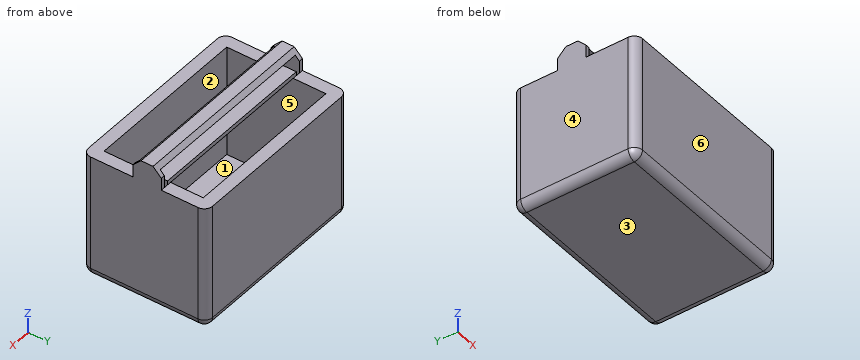
```python
from build123d import *

# Parameters (mm, degrees)
F0_W         = 116.5109202266
F0_H         = 75.9218987077
F1_DEPTH     = 76.2
F2_T         = -7.62
F3_W         = 116.5109202266
F3_H         = 17.5204388797
F4_DEPTH     = 12.7
F5_T         = -2.54
F6_R         = 5.08
F7_R         = 5.08
F8_R         = 5.08
F9_T1_DEPTH  = 66.04
F9_T3_DEPTH  = 106.3509202266
F9_T5_DEPTH  = 83.5418987077
F9_S9_W      = 5.08
F9_S9_H      = 5.08
F9_T10_DEPTH = 5.08
F9_T14_ANGLE = 90
F9_T16_ANGLE = 90
F10_T1_DEPTH = 142.6392193843
F11_T1_DEPTH = 142.6392193843


# Not quite as in the source:
# - a fillet or chamfer that OpenCascade refuses, or shapes differently, is made with other operations: its cross-section is extruded or revolved along the edge and cut away or added
# - a shell that OpenCascade refuses in one call is made with other operations: the cavity is built on its own and cut out


with BuildPart() as f1:
    # F0 (on Front) → F1 (new body)
    with BuildSketch(Plane.XZ):
        with Locations((6.8621747196, 17.2284292057)):
            Rectangle(F0_W, F0_H)
    extrude(amount=F1_DEPTH)

    # F2
    f2_openings = [f1.faces().sort_by_distance(p)[0] for p in [
        (6.862175, -38.1, 55.189379),
    ]]
    offset(amount=F2_T, openings=f2_openings)

    # F3 (on face) → F4 (join)
    with BuildSketch(Plane.XY.offset(55.1893785596)):
        with Locations((6.8621747196, -36.5009140223)):
            Rectangle(F3_W, F3_H)
    extrude(amount=F4_DEPTH)

    # F5: a shell. OpenCascade refuses it in one call, so the cavity is built on its own and cut out:
    # the body offset inwards by the wall thickness, plus a prism from it out through each open face.
    f5_core = offset(f1.part, amount=F5_T, kind=Kind.INTERSECTION, mode=Mode.PRIVATE)
    f5_exits = [f5_core.faces().sort_by_distance(p)[0] for p in [
        (6.862175, -42.721133, 61.352079),
        (6.862175, -30.280695, 61.352079),
    ]]
    add(f5_core, mode=Mode.SUBTRACT)
    extrude(f5_exits, amount=-F5_T, mode=Mode.SUBTRACT)

    # F6
    f6_edges = [f1.edges().sort_by_distance(p)[0] for p in [
        (65.117635, 0, 17.228429),
    ]]
    fillet(f6_edges, radius=F6_R)

    # F7
    f7_edges = [f1.edges().sort_by_distance(p)[0] for p in [
        (4.322175, 0, -20.73252),
        (-51.393285, 0, 17.228429),
    ]]
    fillet(f7_edges, radius=F7_R)

    # F8
    f8_edges = [f1.edges().sort_by_distance(p)[0] for p in [
        (-51.393285, -76.2, 17.228429),
    ]]
    fillet(f8_edges, radius=F8_R)

    # F9: fillet of radius 5.08 on 1 edges, made by hand

    # F9_s2 → F9_t1 (cut)
    with BuildSketch(Plane.XZ.offset(5.08)):
        with BuildLine():
            ThreePointArc((-51.3932853937, -15.6525201482), (-49.9053878421, -19.2446225966), (-46.3132853937, -20.7325201482))
            Line((-46.3132853937, -20.7325201482), (-51.3932853937, -20.7325201482))
            Line((-51.3932853937, -20.7325201482), (-51.3932853937, -15.6525201482))
        make_face()
    extrude(amount=F9_T1_DEPTH, mode=Mode.SUBTRACT)

    # F9_s4 → F9_t3 (cut)
    with BuildSketch(Plane.YZ.offset(-46.3132853937)):
        with BuildLine():
            ThreePointArc((-71.12, -20.7325201482), (-74.7121024484, -19.2446225966), (-76.2, -15.6525201482))
            Line((-76.2, -15.6525201482), (-76.2, -20.7325201482))
            Line((-76.2, -20.7325201482), (-71.12, -20.7325201482))
        make_face()
    extrude(amount=F9_T3_DEPTH, mode=Mode.SUBTRACT)

    # F9_s6 → F9_t5 (cut)
    with BuildSketch(Plane.XY.offset(-15.6525201482)):
        with BuildLine():
            ThreePointArc((60.0376348329, -76.2), (63.6297372813, -74.7121024484), (65.1176348329, -71.12))
            Line((65.1176348329, -71.12), (65.1176348329, -76.2))
            Line((65.1176348329, -76.2), (60.0376348329, -76.2))
        make_face()
    extrude(amount=F9_T5_DEPTH, mode=Mode.SUBTRACT)


with BuildPart() as f9_tool8:
    # F9_s9 → F9_t10 (new body)
    with BuildSketch(Plane.YZ.offset(-46.3132853937)):
        with Locations((-2.54, -18.1925201482)):
            Rectangle(F9_S9_W, F9_S9_H)
    extrude(amount=-F9_T10_DEPTH)

    # F9_s11 → F9_t12 (revolve, cut)
    with BuildSketch(Plane(origin=(-46.3132853937, -5.08, -15.6525201482), x_dir=(0, -0.7071067812, 0.7071067812), z_dir=(0, -0.7071067812, -0.7071067812))):
        with BuildLine():
            ThreePointArc((0, -5.08), (5.08, 0), (0, 5.08))
            Line((0, 5.08), (0, -5.08))
        make_face()
    revolve(axis=Axis((-46.3132853937, -5.08, -15.6525201482), (-1, 0, 0)), mode=Mode.SUBTRACT)


with BuildPart() as f1_1:
    add(f1.part)

    # F9_t7: cut F9_tool8
    add(f9_tool8.part, mode=Mode.SUBTRACT)

    # F9_s13 → F9_t14 (revolve, cut)
    with BuildSketch(Plane.XZ.offset(71.12)):
        with BuildLine():
            ThreePointArc((-46.3132853937, -20.7325201482), (-49.9053878421, -19.2446225966), (-51.3932853937, -15.6525201482))
            Line((-51.3932853937, -15.6525201482), (-51.3932853937, -20.7325201482))
            Line((-51.3932853937, -20.7325201482), (-46.3132853937, -20.7325201482))
        make_face()
    revolve(axis=Axis((-46.3132853937, -71.12, -20.7325201482), (0, 0, 1)), revolution_arc=F9_T14_ANGLE, mode=Mode.SUBTRACT)

    # F9_s15 → F9_t16 (revolve, cut)
    with BuildSketch(Plane.XY.offset(-15.6525201482)):
        with BuildLine():
            ThreePointArc((60.0376348329, -76.2), (63.6297372813, -74.7121024484), (65.1176348329, -71.12))
            Line((65.1176348329, -71.12), (65.1176348329, -76.2))
            Line((65.1176348329, -76.2), (60.0376348329, -76.2))
        make_face()
    revolve(axis=Axis((60.0376348329, -76.2, -15.6525201482), (0, 1, 0)), revolution_arc=F9_T16_ANGLE, mode=Mode.SUBTRACT)

    # F10: chamfer of 5.08 on 1 edges, made by hand

    # F10_s2 → F10_t1 (cut)
    with BuildSketch(Plane.YZ.offset(-64.4574349726)):
        Polygon((-45.2611334622, 62.8093785596), (-40.1811334622, 67.8893785596), (-45.2611334622, 67.8893785596), align=None)
    extrude(amount=F10_T1_DEPTH, mode=Mode.SUBTRACT)

    # F11: chamfer of 5.08 on 1 edges, made by hand

    # F11_s2 → F11_t1 (cut)
    with BuildSketch(Plane.YZ.offset(-64.4574349726)):
        Polygon((-32.8206945825, 67.8893785596), (-27.7406945825, 62.8093785596), (-27.7406945825, 67.8893785596), align=None)
    extrude(amount=F11_T1_DEPTH, mode=Mode.SUBTRACT)


solid = f1_1.part
```
Model file for the job. Use its own axes, mm. Face numbers are marked on the shaded views. A direction names the side the tool comes from. Coordinates: 2 decimals unless noted, no trailing zeros. Loops run counter-clockwise (first coordinate to the right, second up) from the corner with the lowest first, then second, coordinate; pieces in that order, holes last. Notation, with made-up numbers: (11.5, 9) - (45.5, 9) arc R24 cw to (45.5, 46) - close; hole circle Ø3 at (67, 11.5). An arc over 180 degrees is marked (long way). Write item = value, one per line. Start each with the question number.
Item 1: Saw through at B-B, the plane x = 9. List the corners of the cut face in (y, z).
Item 2: Saw through at A-A, the plane z = -6. List the corners of the cut face in (x, y), then the cut area to 3 significant figures.
Item 3: 3-axis set-ups, long thin cutter, end or side, ignore diameter. For the marked faces 1, 2 and 3: which of +Z, -Z, +X, -X, +Y, -Y reach the whole face in a straight line?
Item 4: Drop flat-ended pins along their axis: pin 1 Ø9.5 at (x, y) = (31, -54.5) entering from +Z; pin 2 Ø0.8 at (x, z) = (62, 54.5) entering from -Y; pin 3 Ø0.8 at (x, z) = (-48, 54.5) entering from +Y. Give the stop position or say it passes through.
Item 5: Wall check: probe 1 along Z at (x, y) = (-12, -36.5); probe 2 along X at (y, z) = (-51, 18); probe 3 along Y at (x, z) = (26, 52). Give the ranges that are in metal, low to high. Write a range as [from, to].
Item 6: Pull direction Y, two halves, no side cores. Call the marked faces 4, 5 and 6: +Y half, -Y half, draft (parallel to the pull), parting line (faces both ways), or undercut.
Item 7: Saw through at C-C, the plane y = -12.5. List the corners of the cut face in (x, z).
Answers:
q1.outline = (-76.2, -15.65) arc R5.08 ccw to (-71.12, -20.73) - (-5.08, -20.73) arc R5.08 ccw to (0, -15.65) - (0, 55.19) - (-7.62, 55.19) - (-7.62, -13.11) - (-68.58, -13.11) - (-68.58, 55.19) - (-76.2, 55.19) - close; (-45.26, 55.19) - (-27.74, 55.19) - (-27.74, 57.73) - (-45.26, 57.73) - close; (-42.72, 65.35) - (-30.28, 65.35) - (-32.82, 67.89) - (-40.18, 67.89) - close; hole (-73.66, -18.19) - (-2.54, -18.19) - (-2.54, 52.65) - (-5.08, 52.65) - (-5.08, -15.65) - (-71.12, -15.65) - (-71.12, 52.65) - (-73.66, 52.65) - close
q2.outline = (-51.39, -71.12) arc R5.08 ccw to (-46.31, -76.2) - (60.04, -76.2) arc R5.08 ccw to (65.12, -71.12) - (65.12, -5.08) arc R5.08 ccw to (60.04, 0) - (-46.31, 0) arc R5.08 ccw to (-51.39, -5.08) - close; (-46.31, -71.12) - (60.04, -71.12) - (60.04, -5.08) - (-46.31, -5.08) - close; hole (-48.85, -73.66) - (62.58, -73.66) - (62.58, -2.54) - (-48.85, -2.54) - close; hole (-43.77, -68.58) - (57.5, -68.58) - (57.5, -7.62) - (-43.77, -7.62) - close
q2.area = 1,780 mm2
q3.face_1 = none
q3.face_2 = +Z
q3.face_3 = -Z, +X, -X, +Y, -Y
q4.pin_1 = -13.11
q4.pin_2 = -75.95
q4.pin_3 = -0.17
q5.probe_1 = [-20.73, -18.19], [-15.65, -13.11], [55.19, 57.73], [65.35, 67.89]
q5.probe_2 = [-51.39, -48.85], [-46.31, -43.77], [57.5, 60.04], [62.58, 65.12]
q5.probe_3 = [-76.2, -73.66], [-71.12, -68.58], [-7.62, -5.08], [-2.54, 0]
q6.face_4 = draft
q6.face_5 = undercut
q6.face_6 = -Y half
q7.outline = (-51.39, -15.65) arc R5.08 ccw to (-46.31, -20.73) - (60.04, -20.73) arc R5.08 ccw to (65.12, -15.65) - (65.12, 55.19) - (57.5, 55.19) - (57.5, -13.11) - (-43.77, -13.11) - (-43.77, 55.19) - (-51.39, 55.19) - close; hole (-48.85, -18.19) - (62.58, -18.19) - (62.58, 52.65) - (60.04, 52.65) - (60.04, -15.65) - (-46.31, -15.65) - (-46.31, 52.65) - (-48.85, 52.65) - close
